Autodesk Inventor part; units mm, degrees
ref_plane "Work Plane2" through (2.8575, 0, 0) normal (0.7071, 0, 0.7071) x (0.7071, 0, -0.7071)
ref_plane "YZ Plane" through (0, 0, 0) normal (1, 0, 0) x (0, 1, 0)
ref_plane "XZ Plane" through (0, 0, 0) normal (0, 1, 0) x (-1, 0, 0)
sketch "Sketch1" plane through (0, 0, 0) normal (0, 1, 0) x (-1, 0, 0)
  circle A0 centre (0, 0) radius 1.5875
  line L0 (0, 0) -> (0, -7.62)
  circle A1 centre (0, -7.62) radius 1.5875
  line L1 (-14.0081, -3.81) -> (-6.6675, -3.81)
  circle A2 centre (10.1981, -3.81) radius 1.5875
  line L2 (10.1981, -3.81) -> (10.1981, -6.35)
  line L3 (10.1981, -6.35) -> (10.1981, -1.27)
  line L4 (0, 1.5875) -> (0, 2.8575)
  line L5 (-1.5875, 0) -> (-2.8575, 0)
  line L6 (0, -9.2075) -> (0, -10.4775)
  line L7 (-1.5875, -7.62) -> (-2.8575, -7.62)
  line L8 (-2.8575, -7.62) -> (-2.8575, 0)
  line L9 (0, 2.8575) -> (-2.8575, 0)
  line L10 (0, 2.8575) -> (3.4925, 1.444)
  line L11 (3.4925, -9.064) -> (0, -10.4775)
  line L12 (-2.8575, -7.62) -> (0, -10.4775)
  line L13 (-2.8575, -3.81) -> (0, -3.81)
  line L14 (3.4925, -3.81) -> (3.4925, -9.064)
  line L15 (3.4925, -3.81) -> (3.4925, 1.444)
  line L16 (10.1981, -3.81) -> (12.7381, -3.81)
  line L17 (12.7381, -3.81) -> (12.7381, -6.35)
  line L18 (12.7381, -6.35) -> (10.1981, -6.35)
  line L19 (12.7381, -3.81) -> (12.7381, -1.27)
  line L20 (12.7381, -1.27) -> (10.1981, -1.27)
  line L21 (12.7381, -6.35) -> (0, -10.4775)
  line L22 (12.7381, -1.27) -> (0, 2.8575)
  line L23 (10.1981, -3.81) -> (12.7381, -3.81)
  line L24 (3.4925, 1.444) -> (3.4925, 1.7258)
  line L25 (3.4925, -9.064) -> (3.4925, -9.3458)
  dimension "d0" = 3.175
  dimension "d1" = 7.62
  dimension "d2" = 3.175
  dimension "d3" = 7.3406
  dimension "d4" = 3.175
  dimension "d7" = 5.08
  dimension "d8" = 1.27
  dimension "d9" = 1.27
  dimension "d10" = 1.27
  dimension "d11" = 1.27
  dimension "d12" = 6.35
  dimension "d44" = 2.54
ref_plane "Work Plane2" through (2.8575, 0, 0) normal (0.7071, 0, 0.7071) x (0.7071, 0, -0.7071)
sketch "Sketch3" plane through (2.8575, 0, 0) normal (0.7071, 0, 0.7071) x (0.7071, 0, -0.7071)
  point P0 (-2.0206, 0)
extrude "Extrusion4" add sketch "Sketch1" along normal blind 1.905 contours A0 L4 L10 L15 L14 L11 L6 A1 L0 | A0 L5 L9 L4 | L0 L13 L8 L5 A0 | L22 L24 L10 | L0 A1 L7 L8 L13 | A1 L6 L12 L7 | L25 L21 L11
extrude "Extrusion5" add sketch "Sketch1" along normal blind 3.81 contours L24 L22 L20 L3 A2 L2 L18 L21 L25 L14 L15 | L19 L16 A2 L3 L20 | L17 L18 L2 A2 L16
extrude "Extrusion6" add sketch "Sketch1" along normal blind 1.905 contours A0 | A1
properties part number "rollertriangle(v3)"
Check sheet for the modelled part. Datum: model origin and axes. Units: mm. A direction names the side the tool comes from. Round coordinates to 2 decimals unless told otherwise and drop trailing zeros. Order: outer loops, then holes, each group sorted by start corner. A loop starts at its lowest first (then second) coordinate and runs counter-clockwise, first axis right, second up. Notation, with made-up numbers: (5, 53.5) - (23, 53.5) arc R6 ccw to (23, 62.5) - close; hole circle Ø7 at (-3.5, -24.5). An arc over 180 degrees is marked (long way). Answer as CSV lines item,"result". Start each with the question number.
1) Depth check by flat-ended pin: pin 1 (0.6 mm diameter, centred on y = 3, z = -2, fed in from +X). Enter the tip coordinate at first touch or a pass-through.
2) Section check A-A (z = -3.81). Record the cut outline in (x, y) (1 decimal), then the cut area to 3 significant figures.
3) Draft check along Z on faces 1 (the face through (1.41, 0.94, 1.45)), 2 (the face through (-12.738, 2, -4)), 3 (the face through (-11.665, 1.878, -3.202)). Enter one of: +Z half, -Z half, draft (parallel to the pull), parting line (faces both ways), or undercut.
4) Tool access check on faces 4 (the face through (1.45, 0.94, -9.03)), 5 (the face through (0, 1.905, -4)). Record the directions out of +Z, -Z, +X, -X, +Y, -Y that give a thin tool (end or side, any length) a straight path to the whole face; none if there is none.
5) Scan lines: probe 1 along X at (y, z) = (2, -3.81); probe 2 along X at (y, z) = (1.15, -3.81); probe 3 along X at (y, z) = (3.6, -6.25). Record each from-to range of solid material in increasing order.
6) Section check D-D (z = -9). Record the cut outline in (x, y) (1 decimal).
Determined:
1,pin 1,"x = -3.49"
2,outline,"(-12.7, 0) - (-11.8, 0) - (-11.8, 3.8) - (-12.7, 3.8) - close; (-8.6, 0) - (2.9, 0) - (2.9, 1.9) - (-3.5, 1.9) - (-3.5, 3.8) - (-8.6, 3.8) - close"
2,area,"35.2 mm^2"
3,face 1,"+Z half"
3,face 2,"draft"
3,face 3,"undercut"
4,face 4,"-Z, +X, +Y, -Y"
4,face 5,"+Z, -Z, +X, +Y"
5,probe 1,"-12.74 to -11.79, -8.61 to -3.49"
5,probe 2,"-12.74 to -11.79, -8.61 to 2.86"
5,probe 3,"-12.74 to -3.49"
6,outline,"(-4.6, 0) - (1.5, 0) - (1.5, 1.9) - (-3.5, 1.9) - (-3.5, 3.8) - (-4.6, 3.8) - close"
